from build123d import *

# Parameters (mm, degrees)
BOSS_EXTRUDE1_DEPTH = 12.7
CUT_EXTRUDE1_REACH  = 78.2
SKETCH3_R           = 3.175
SKETCH4_W           = 28.507373457
SKETCH4_H           = 9.150354521
CUT_EXTRUDE2_DEPTH  = 4.52374
SKETCH5_R           = 3.175
CUT_EXTRUDE3_DEPTH  = 7.35


with BuildPart() as part:
    # Sketch2 → Boss-Extrude1 (new body, symmetric)
    with BuildSketch(Plane.XY):
        with BuildLine():
            Line((-38.1, 0), (38.1, 0))
            Line((38.1, 0), (38.1, 101.6))
            Line((38.1, 101.6), (34.925, 101.6))
            ThreePointArc((34.925, 101.6), (32.67993597, 100.67006403), (31.75, 98.425))
            Line((31.75, 98.425), (31.75, 9.525))
            ThreePointArc((31.75, 9.525), (30.82006403, 7.27993597), (28.575, 6.35))
            Line((28.575, 6.35), (-34.925, 6.35))
            ThreePointArc((-34.925, 6.35), (-37.17006403, 5.42006403), (-38.1, 3.175))
            Line((-38.1, 3.175), (-38.1, 0))
        make_face()
    extrude(amount=BOSS_EXTRUDE1_DEPTH, both=True)

    # Sketch3 → Cut-Extrude1 (cut, up to next)
    with BuildSketch(Plane(origin=(38.1, 0, 0), x_dir=(0, 0, -1), z_dir=(1, 0, 0)), mode=Mode.PRIVATE) as cut_extrude1_sk1:
        with Locations((0, 76.2)):
            Circle(SKETCH3_R)
    cut_extrude1_tool1 = extrude(cut_extrude1_sk1.sketch, amount=-CUT_EXTRUDE1_REACH, mode=Mode.PRIVATE) & part.part
    add(cut_extrude1_tool1.solids().sort_by_distance((38.1, 76.2, 0))[0], mode=Mode.SUBTRACT)
    # Sketch3 → Cut-Extrude1 (cut, up to next)
    with BuildSketch(Plane(origin=(38.1, 0, 0), x_dir=(0, 0, -1), z_dir=(1, 0, 0)), mode=Mode.PRIVATE) as cut_extrude1_sk2:
        with Locations((0, 25.4)):
            Circle(SKETCH3_R)
    cut_extrude1_tool2 = extrude(cut_extrude1_sk2.sketch, amount=-CUT_EXTRUDE1_REACH, mode=Mode.PRIVATE) & part.part
    add(cut_extrude1_tool2.solids().sort_by_distance((38.1, 25.4, 0))[0], mode=Mode.SUBTRACT)

    # Sketch4 → Cut-Extrude2 (cut)
    with BuildSketch(Plane.ZY.offset(38.1)):
        with Locations((1.553686728, 4.575177261)):
            Rectangle(SKETCH4_W, SKETCH4_H)
    extrude(amount=-CUT_EXTRUDE2_DEPTH, mode=Mode.SUBTRACT)

    # Sketch5 → Cut-Extrude3 (cut, through all)
    with BuildSketch(Plane(origin=(0, 6.35, 0), x_dir=(1, 0, 0), z_dir=(0, 1, 0))):
        with Locations((-1.82626, 0)):
            Circle(SKETCH5_R)
        with Locations((-20.87626, 0)):
            Circle(SKETCH5_R)
    extrude(amount=-CUT_EXTRUDE3_DEPTH, mode=Mode.SUBTRACT)


solid = part.part
The model under review builds one solid part; all positions refer to its coordinate system, in mm. A direction names the side the tool comes from. Round coordinates to 2 decimals unless told otherwise and drop trailing zeros. Order: outer loops, then holes, each group sorted by start corner. A loop starts at its lowest first (then second) coordinate and runs counter-clockwise, first axis right, second up. Notation, with made-up numbers: (-2.5, 24) -> (30.5, 24) arc R24 cw to (30.5, 51) -> close; hole circle Ø6 at (34, -11). An arc over 180 degrees is marked (long way). Use CSV: the item, a comma, the result in double quotes. Start each with the question number.
(1) Mouldability with a two-part tool opening along Y and no side actions: class faces 3 (the face through (-2, 6.35, -5)), 4 (the face through (2, 0, 0)), 5 (the face through (34.969, 78.877, -1.707)) as pulls with the +Y half, pulls with the -Y half, needs draft (parallel to the pull), parting line crosses it, or undercut.
(2) Wall thickness on probe 1 along X at (y, z) = (2.75, 0); probe 2 along Y at (x, z) = (35.75, 0) (3 decimals); probe 3 along Z at (x, y) = (36, 76): over which ranges is each line inside the solid? List them lowest first. Write a range as from..to.
(3) Tool access review of faces 1 (the face through (31.75, 55, 0)), 2 (the face through (37, 101.6, 0)): name each direction out of +Z, -Z, +X, -X, +Y, -Y from which nothing blocks a thin tool from reaching the whole face with its end or side.
(4) Consider section B-B on z = -6.25. Write out the cut boundary in (x, y) (3 decimals), and give its area (3 significant figures).
(5) Consider section C-C on x = 26. Write out the cut boundary in (y, z).
(6) Consider section A-A on y = 76.2. Write out the cut boundary in (x, z) (3 decimals), and give its area (3 significant figures).
(7) Insertion check: pin 1 (8.5 mm diameter, centred on y = 25.4, z = 0, fed in from -X); pin 2 (6 mm diameter, centred on x = 24.5, z = -4.5, fed in from -Y). Each pin has a flat end and moves straight along its axis. Give the tip position at first contact, or say it passes through.
Responses:
1,face 3,"pulls with the +Y half"
1,face 4,"pulls with the -Y half"
1,face 5,"undercut"
2,probe 1,"-33.58..-24.05, -17.7..-5, 1.35..38.1"
2,probe 2,"0..22.225, 28.575..73.025, 79.375..101.6"
2,probe 3,"-12.7..-3.17, 3.17..12.7"
3,face 1,"+Z, -Z, -X, +Y"
3,face 2,"+Z, -Z, +X, -X, +Y"
4,outline,"(-33.576, 0) -> (38.1, 0) -> (38.1, 101.6) -> (34.925, 101.6) arc R3.175 ccw to (31.75, 98.425) -> (31.75, 9.525) arc R3.175 cw to (28.575, 6.35) -> (-33.576, 6.35) -> close"
4,area,"1,060 mm²"
5,outline,"(0, -12.7) -> (6.35, -12.7) -> (6.35, 12.7) -> (0, 12.7) -> close"
6,outline,"(31.75, -12.7) -> (38.1, -12.7) -> (38.1, -3.175) -> (31.75, -3.175) -> close; (31.75, 3.175) -> (38.1, 3.175) -> (38.1, 12.7) -> (31.75, 12.7) -> close"
6,area,"121 mm²"
7,pin 1,"x = 31.75"
7,pin 2,"y = 0"
